Source: CAD feature listing. Evaluate the final solid. Frame: model axes, mm. Face numbers are marked on the shaded views. Coordinates: 2 decimals unless noted, no trailing zeros. Write each loop counter-clockwise with the first axis right and the second up, starting at its lowest first coordinate (ties: lowest second). Pieces come first, ordered by that corner, then holes. Notation, with made-up numbers: M -32.5,6 L 12.5,6 A22 cw 12.5,37 Z; hole C 80,-1 d2. An arc over 180 degrees is marked long. Answer as CSV lines item,"result". Start each with the question number.
1. Contact query for flat-ended pins moving along their axis: pin 1 Ø3.5 at (x, z) = (7.5, 8) entering from -Y; pin 2 Ø6 at (x, z) = (8.5, 14) entering from +Y; pin 3 Ø3 at (y, z) = (7, 6.5) entering from -X; pin 4 Ø1 at (x, z) = (14.5, 33) entering from -Y. Output: stop coordinate, or through.
2. Mould query, pull axis Y, two halves, no side actions, for the marked faces 1, 2 and 3. Classes: pulls with the +Y half, pulls with the -Y half, needs draft (parallel to the pull), parting line crosses it, or undercut.
3. Section C-C on z = 8. Return the cut outline in (x, y).
4. Section B-B on x = 7.5. Return the cut outline in (y, z).
5. Section D-D on z = 13. Return the cut outline in (x, y).
6. Line query: probe 1 along Y at (x, z) = (13.95, 28); probe 2 along Y at (x, z) = (14.55, 9); probe 3 along X at (y, z) = (36, 18.5). Output: solid intervals per line, ascending. Write a range as [from, to].
7. Section A-A on z = 18. Return the cut outline in (x, y).
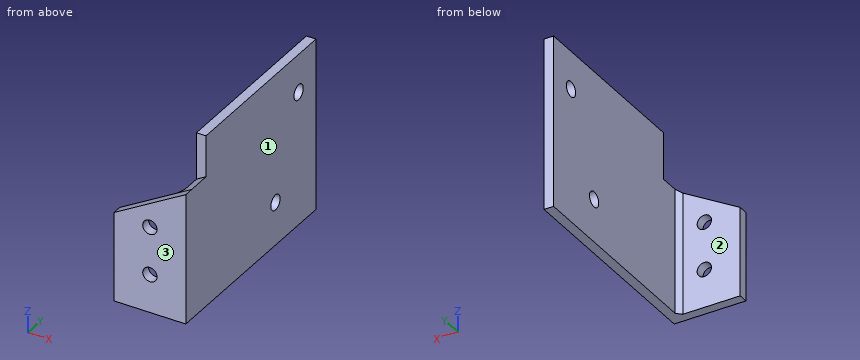
```python
from build123d import *

# Parameters (mm, degrees)
EXTRUDE_2_DEPTH     = 36
CUT_EXTRUDE_4_REACH = 61.548
SKETCH_7_R          = 1.5
CHAMFER_2_SIZE      = 1
CUT_EXTRUDE_5_REACH = 61.548
SKETCH_8_R          = 1.6
CUT_EXTRUDE_6_REACH = 60.052
CUT_EXTRUDE_8_DEPTH = 5


with BuildPart() as part:
    # ｽｹｯﾁ6 → ﾎﾞｽ - 押し出し2 (new body)
    with BuildSketch(Plane.XY):
        Polygon((0, 0), (15, 0), (15, 45), (13, 45), (13, 2), (0, 2), align=None)
    extrude(amount=EXTRUDE_2_DEPTH)

    # ｽｹｯﾁ7 → ｶｯﾄ - 押し出し4 (cut, up to next)
    with BuildSketch(Plane.XZ, mode=Mode.PRIVATE) as cut_extrude_4_sk1:
        with Locations(Location((7.5, 18, 0), (0, 0, 270))):
            Circle(SKETCH_7_R)
    cut_extrude_4_tool1 = extrude(cut_extrude_4_sk1.sketch, amount=-CUT_EXTRUDE_4_REACH, mode=Mode.PRIVATE) & part.part
    # ｽｹｯﾁ7 → ｶｯﾄ - 押し出し4 (cut, up to next)
    with BuildSketch(Plane.XZ, mode=Mode.PRIVATE) as cut_extrude_4_sk2:
        with Locations(Location((7.5, 8, 0), (0, 0, 270))):
            Circle(SKETCH_7_R)
    cut_extrude_4_tool2 = extrude(cut_extrude_4_sk2.sketch, amount=-CUT_EXTRUDE_4_REACH, mode=Mode.PRIVATE) & part.part
    add(cut_extrude_4_tool1.solids().sort_by_distance((7.5, 0, 18))[0], mode=Mode.SUBTRACT)
    add(cut_extrude_4_tool2.solids().sort_by_distance((7.5, 0, 8))[0], mode=Mode.SUBTRACT)

    # 面取り2
    chamfer_2_edges = [part.edges().sort_by_distance(p)[0] for p in [
        (13, 2, 18),
    ]]
    chamfer(chamfer_2_edges, length=CHAMFER_2_SIZE)

    # ｽｹｯﾁ8 → ｶｯﾄ - 押し出し5 (cut, up to next)
    with BuildSketch(Plane(origin=(15, 0, 0), x_dir=(0, 0, -1), z_dir=(1, 0, 0)), mode=Mode.PRIVATE) as cut_extrude_5_sk1:
        with Locations((-28, 39)):
            Circle(SKETCH_8_R)
    cut_extrude_5_tool1 = extrude(cut_extrude_5_sk1.sketch, amount=-CUT_EXTRUDE_5_REACH, mode=Mode.PRIVATE) & part.part
    # ｽｹｯﾁ8 → ｶｯﾄ - 押し出し5 (cut, up to next)
    with BuildSketch(Plane(origin=(15, 0, 0), x_dir=(0, 0, -1), z_dir=(1, 0, 0)), mode=Mode.PRIVATE) as cut_extrude_5_sk2:
        with Locations((-9, 31)):
            Circle(SKETCH_8_R)
    cut_extrude_5_tool2 = extrude(cut_extrude_5_sk2.sketch, amount=-CUT_EXTRUDE_5_REACH, mode=Mode.PRIVATE) & part.part
    add(cut_extrude_5_tool1.solids().sort_by_distance((15, 39, 28))[0], mode=Mode.SUBTRACT)
    add(cut_extrude_5_tool2.solids().sort_by_distance((15, 31, 9))[0], mode=Mode.SUBTRACT)

    # ｽｹｯﾁ9 → ｶｯﾄ - 押し出し6 (cut, up to next)
    with BuildSketch(Plane(origin=(0, 2, 0), x_dir=(1, 0, 0), z_dir=(0, 1, 0)), mode=Mode.PRIVATE) as cut_extrude_6_sk1:
        Polygon((0, -36), (30, -36), (0, -18.679491924), align=None)
    cut_extrude_6_tool1 = extrude(cut_extrude_6_sk1.sketch, amount=-CUT_EXTRUDE_6_REACH, mode=Mode.PRIVATE) & part.part
    add(cut_extrude_6_tool1.solids().sort_by_distance((10, 2, 30.226497))[0], mode=Mode.SUBTRACT)

    # ｽｹｯﾁ11 → ｶｯﾄ - 押し出し8 (cut)
    with BuildSketch(Plane.XZ.offset(-2)):
        Polygon((12, 25.607695155), (15, 27.339745962), (15, 36), (12, 36), align=None)
    extrude(amount=-CUT_EXTRUDE_8_DEPTH, mode=Mode.SUBTRACT)


solid = part.part
```
Values:
1,pin 1,"y = 0"
1,pin 2,"y = 2"
1,pin 3,"x = 13"
1,pin 4,"y = 7"
2,face 1,"needs draft"
2,face 2,"pulls with the +Y half"
2,face 3,"pulls with the -Y half"
3,outline,"M 0,0 L 6,0 L 6,2 L 0,2 Z; M 9,0 L 15,0 L 15,29.75 L 13,29.75 L 13,3 L 12,2 L 9,2 Z; M 13,32.25 L 15,32.25 L 15,45 L 13,45 Z"
4,outline,"M 0,0 L 2,0 L 2,6.5 L 0,6.5 Z; M 0,9.5 L 2,9.5 L 2,16.5 L 0,16.5 Z; M 0,19.5 L 2,19.5 L 2,23.01 L 0,23.01 Z"
5,outline,"M 0,0 L 15,0 L 15,45 L 13,45 L 13,3 L 12,2 L 0,2 Z"
6,probe 1,"[7, 37.4], [40.6, 45]"
6,probe 2,"[0, 29.4], [32.6, 45]"
6,probe 3,"[13, 15]"
7,outline,"M 0,0 L 6,0 L 6,2 L 0,2 Z; M 9,0 L 15,0 L 15,45 L 13,45 L 13,3 L 12,2 L 9,2 Z"
